Geometry check sheet. Reference: the model listing, model coordinates, mm. Face numbers are marked on the shaded views. Give positions to 0.01 mm unless a question says otherwise; leave off trailing zeros. Order: outer loops, then holes, each group sorted by start corner. A loop starts at its lowest first (then second) coordinate and runs counter-clockwise, first axis right, second up. Notation, with made-up numbers: M -24.5,71 L 0.5,71 A26 ccw 0.5,92 Z; hole C -24,33 d5. An arc over 180 degrees is marked long. Answer as CSV lines item,"result".
from build123d import *

# Parameters (mm, degrees)
SKETCH1_W           = 212
SKETCH1_H           = 125
BOSS_EXTRUDE1_DEPTH = 6.6
SKETCH2_W           = 182
SKETCH2_H           = 121
CUT_EXTRUDE1_DEPTH  = 1.2
CUT_EXTRUDE2_DEPTH  = 131.2
CUT_EXTRUDE3_DEPTH  = 131.2
CUT_EXTRUDE4_DEPTH  = 221.2
CUT_EXTRUDE5_DEPTH  = 221.2
FILLET1_R           = 3
SKETCH7_R           = 2.5
CUT_EXTRUDE6_DEPTH  = 6
SKETCH8_R           = 3.5
CUT_EXTRUDE7_DEPTH  = 1
SKETCH9_R           = 2
CUT_EXTRUDE8_DEPTH  = 5
SKETCH10_R          = 0.6
CUT_EXTRUDE9_DEPTH  = 1.5
CHAMFER1_SIZE       = 0.5
CUT_EXTRUDE10_DEPTH = 1.5
CUT_EXTRUDE11_DEPTH = 1.5


with BuildPart() as part:
    # Sketch1 → Boss-Extrude1 (new body)
    with BuildSketch(Plane(origin=(0, 0, 0), x_dir=(1, 0, 0), z_dir=(0, 1, 0))):
        with Locations((-26.64556962, -19.170886076)):
            Rectangle(SKETCH1_W, SKETCH1_H)
    extrude(amount=BOSS_EXTRUDE1_DEPTH)

    # Sketch2 → Cut-Extrude1 (cut)
    with BuildSketch(Plane(origin=(0, 6.6, 0), x_dir=(1, 0, 0), z_dir=(0, 1, 0))):
        with Locations((-26.64556962, -19.170886076)):
            Rectangle(SKETCH2_W, SKETCH2_H)
    extrude(amount=-CUT_EXTRUDE1_DEPTH, mode=Mode.SUBTRACT)

    # Sketch3 → Cut-Extrude2 (cut)
    with BuildSketch(Plane.XY.offset(81.670886076)):
        Polygon((-132.64556962, 5.6), (-130.64556962, 0), (-132.64556962, 0), align=None)
    extrude(amount=-CUT_EXTRUDE2_DEPTH, mode=Mode.SUBTRACT)

    # Sketch4 → Cut-Extrude3 (cut)
    with BuildSketch(Plane.XY.offset(81.670886076)):
        Polygon((79.35443038, 5.6), (77.35443038, 0), (79.35443038, 0), align=None)
    extrude(amount=-CUT_EXTRUDE3_DEPTH, mode=Mode.SUBTRACT)

    # Sketch5 → Cut-Extrude4 (cut)
    with BuildSketch(Plane(origin=(79.35443038, 0, 0), x_dir=(0, 0, -1), z_dir=(1, 0, 0))):
        Polygon((-81.670886076, 5.6), (-79.670886076, 0), (-81.670886076, 0), align=None)
    extrude(amount=-CUT_EXTRUDE4_DEPTH, mode=Mode.SUBTRACT)

    # Sketch6 → Cut-Extrude5 (cut)
    with BuildSketch(Plane(origin=(79.35443038, 0, 0), x_dir=(0, 0, -1), z_dir=(1, 0, 0))):
        Polygon((43.329113924, 5.6), (41.329113924, 0), (43.329113924, 0), align=None)
    extrude(amount=-CUT_EXTRUDE5_DEPTH, mode=Mode.SUBTRACT)

    # Fillet1
    # the kernel refuses this fillet: 3 mm, written as the material it takes off along each edge
    with BuildSketch(Plane(origin=(75.220284038, -5.975609756, 77.536739734), x_dir=(0.1072201272408216, 0.30021635627431204, -0.9478259248088952), z_dir=(0.3187883565316692, 0.8926073982886735, 0.31878835653166915)), Plane(origin=(75.220284038, -5.975609756, -39.194967583), x_dir=(-0.9478259248088952, 0.30021635627431126, -0.10722012724082396), z_dir=(0.31878835653166926, 0.892607398288674, -0.3187883565316682))) as fillet1_piece_1:
        with BuildLine():
            CenterArc((FILLET1_R * 0.892607398289, FILLET1_R), FILLET1_R, 186.495326626, 83.504673374)
            Line((-FILLET1_R * 0.100973687589, FILLET1_R * 0.886877828054), (0, 0))
            Line((0, 0), (FILLET1_R * 0.892607398289, 0))
        make_face()
    extrude(amount=19.662865831, mode=Mode.SUBTRACT)
    with BuildSketch(Plane(origin=(-128.511423279, -5.975609756, 77.536739734), x_dir=(-0.10722012724082589, 0.30021635627431054, -0.947825924808895), z_dir=(-0.3187883565316692, 0.8926073982886735, 0.31878835653166926)), Plane(origin=(-128.511423279, -5.975609756, -39.194967583), x_dir=(0.9478259248088952, 0.30021635627431037, -0.10722012724082654), z_dir=(-0.31878835653166926, 0.892607398288674, -0.3187883565316681))) as fillet1_piece_2:
        with BuildLine():
            CenterArc((FILLET1_R * 0.892607398289, -FILLET1_R), FILLET1_R, 90, 83.504673374)
            Line((-FILLET1_R * 0.100973687589, -FILLET1_R * 0.886877828054), (0, 0))
            Line((0, 0), (FILLET1_R * 0.892607398289, 0))
        make_face()
    extrude(amount=19.662865831, mode=Mode.SUBTRACT)
    with BuildSketch(Plane(origin=(-132.64556962, -1.9, -43.329113924), x_dir=(1, 0, 0), z_dir=(0, 1, 0)), Plane(origin=(-132.64556962, -1.9, 81.670886076), x_dir=(0, 0, -1), z_dir=(0, 1, 0))) as fillet1_piece_3:
        with BuildLine():
            CenterArc((FILLET1_R, -FILLET1_R), FILLET1_R, 90, 90)
            Line((0, -FILLET1_R), (0, 0))
            Line((0, 0), (FILLET1_R, 0))
        make_face()
    extrude(amount=16, mode=Mode.SUBTRACT)
    with BuildSketch(Plane(origin=(79.35443038, -1.9, -43.329113924), x_dir=(-1, 0, 0), z_dir=(0, 1, 0)), Plane(origin=(79.35443038, -1.9, 81.670886076), x_dir=(0, 0, -1), z_dir=(0, 1, 0))) as fillet1_piece_4:
        with BuildLine():
            CenterArc((FILLET1_R, FILLET1_R), FILLET1_R, 180, 90)
            Line((0, FILLET1_R), (0, 0))
            Line((0, 0), (FILLET1_R, 0))
        make_face()
    extrude(amount=16, mode=Mode.SUBTRACT)

    # Sketch7 → Cut-Extrude6 (cut)
    with BuildSketch(Plane.XZ):
        with Locations(Location((-125.64556962, -36.329113924, 0), (0, 0, 270))):
            Circle(SKETCH7_R)
    extrude(amount=-CUT_EXTRUDE6_DEPTH, mode=Mode.SUBTRACT)

    # Sketch8 → Cut-Extrude7 (cut)
    with BuildSketch(Plane.XZ):
        with Locations(Location((-125.64556962, -36.329113924, 0), (0, 0, 270))):
            Circle(SKETCH8_R)
    extrude(amount=-CUT_EXTRUDE7_DEPTH, mode=Mode.SUBTRACT)

    # Sketch9 → Cut-Extrude8 (cut)
    with BuildSketch(Plane(origin=(0, 6.6, 0), x_dir=(1, 0, 0), z_dir=(0, 1, 0))):
        with Locations(Location((72.241534247, 33.329113924, 0), (0, 0, 270))):
            Circle(SKETCH9_R)
    extrude(amount=-CUT_EXTRUDE8_DEPTH, mode=Mode.SUBTRACT)

    # Sketch10 → Cut-Extrude9 (cut)
    with BuildSketch(Plane(origin=(0, 6.6, 0), x_dir=(1, 0, 0), z_dir=(0, 1, 0))):
        with Locations(Location((-121.14556962, 39.465683386, 0), (0, 0, 270))):
            Circle(SKETCH10_R)
        with Locations(Location((-121.157311089, 35.420585215, 0), (0, 0, 270))):
            Circle(SKETCH10_R)
    extrude(amount=-CUT_EXTRUDE9_DEPTH, mode=Mode.SUBTRACT)

    # Chamfer1
    chamfer1_edges = [part.edges().sort_by_distance(p)[0] for p in [
        (-132.64556962, 6.6, 19.170886076),
        (-26.64556962, 6.6, -43.329113924),
        (-26.64556962, 6.6, 81.670886076),
        (79.35443038, 6.6, 19.170886076),
        (78.475750723, 6.6, -42.450434268),
        (78.475750723, 6.6, 80.79220642),
        (-131.766889964, 6.6, 80.79220642),
        (-131.766889964, 6.6, -42.450434268),
    ]]
    chamfer(chamfer1_edges, length=CHAMFER1_SIZE)

    # Sketch11 → Cut-Extrude10 (cut)
    with BuildSketch(Plane(origin=(0, 6.6, 0), x_dir=(1, 0, 0), z_dir=(0, 1, 0))):
        Polygon((-132.14556962, -19.170886076), (-132.14556962, -39.170886076), (-130.14556962, -37.170886076), (-130.14556962, -1.170886076), (-132.14556962, 0.829113924), align=None)
    extrude(amount=-CUT_EXTRUDE10_DEPTH, mode=Mode.SUBTRACT)

    # Sketch12 → Cut-Extrude11 (cut)
    with BuildSketch(Plane(origin=(0, 6.6, 0), x_dir=(1, 0, 0), z_dir=(0, 1, 0))):
        Polygon((78.85443038, -19.170886076), (78.85443038, 0.829113924), (76.85443038, -1.170886076), (76.85443038, -37.170886076), (78.85443038, -39.170886076), align=None)
    extrude(amount=-CUT_EXTRUDE11_DEPTH, mode=Mode.SUBTRACT)


solid = part.part
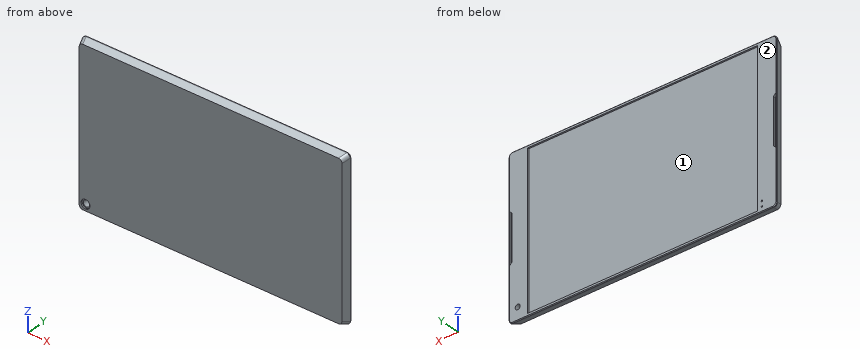
(1) Draft check along Z on the marked faces 1 and 2. Enter one of: +Z half, -Z half, draft (parallel to the pull), parting line (faces both ways), or undercut.
The answers:
face 1,"undercut"
face 2,"draft"
(2) Section check A-A on z = 9. Enter the section's corners in (x, y).
The answers:
outline,"M -132.65,5.6 L -130.65,0 L 77.35,0 L 79.35,5.6 L 79.35,6.1 L 78.85,6.6 L 78.85,5.1 L 76.85,5.1 L 76.85,6.6 L 64.35,6.6 L 64.35,5.4 L -117.65,5.4 L -117.65,6.6 L -130.15,6.6 L -130.15,5.1 L -132.15,5.1 L -132.15,6.6 L -132.65,6.1 Z"
(3) Material ranges on line 1 (X direction, y = 5.5, z = 26); line 2 (X direction, y = 6, z = 43.5); line 3 (Y direction, x = -52.5, z = 57), recorded low to high.
The answers:
line 1,"x = -132.61 to -132.15, -130.15 to -117.65, 64.35 to 76.85, 78.85 to 79.32"
line 2,"x = -132.65 to -117.65, 64.35 to 79.35"
line 3,"y = 0 to 5.4"
(4) Gauge pin test, flat ends, axial feed: P1, Ø0.6, axis at x = -121, z = -39.5, coming from the +Y side; P2, Ø1.2, axis at x = 72, z = -34, coming from the +Y side; P3, Ø4, axis at x = 28.5, z = -15.5, coming from the +Y side. Record the tip position at first contact, or that the pin passes through.
The answers:
P1,"stops at y = 5.1"
P2,"stops at y = 1.6"
P3,"stops at y = 5.4"
(5) Section check D-D on z = -9.5. Enter the section's corners in (x, y).
The answers:
outline,"M -132.65,5.6 L -130.65,0 L 77.35,0 L 79.35,5.6 L 79.35,6.1 L 78.85,6.6 L 64.35,6.6 L 64.35,5.4 L -117.65,5.4 L -117.65,6.6 L -132.15,6.6 L -132.65,6.1 Z"
(6) Section check B-B on x = 57.5. Enter the section's corners in (y, z).
The answers:
outline,"M 0,-41.33 L 5.6,-43.33 L 6.1,-43.33 L 6.6,-42.83 L 6.6,-41.33 L 5.4,-41.33 L 5.4,79.67 L 6.6,79.67 L 6.6,81.17 L 6.1,81.67 L 5.6,81.67 L 0,79.67 Z"
(7) Section check C-C on y = 3.25. State how many separate pieces and enclosed holes the cut face has, then the cut area to 3 significant figures.
The answers:
separate pieces,"1"
enclosed holes,"2"
area,"25,900 mm2"
